from build123d import *

# Parameters (mm, degrees)
SKETCH2_R           = 17.5
SKETCH2_R_2         = 1.475
SKETCH2_R_3         = 4
BOSS_EXTRUDE1_DEPTH = 2.5
SKETCH3_R           = 7.5
SKETCH3_R_2         = 4
BOSS_EXTRUDE2_DEPTH = 10
FILLET1_R           = 1
SKETCH7_R           = 2.153442821
CUT_EXTRUDE7_DEPTH  = 5
CIRPATTERN2_COUNT   = 4


with BuildPart() as part:
    # Sketch2 → Boss-Extrude1 (new body)
    with BuildSketch(Plane(origin=(0, 0, 0), x_dir=(1, 0, 0), z_dir=(0, 1, 0))):
        with Locations(Location((0, 0, 0), (0, 0, 270))):
            Circle(SKETCH2_R)
        with Locations(Location((-12, 0, 0), (0, 0, 270))):
            Circle(SKETCH2_R_2, mode=Mode.SUBTRACT)
        with Locations(Location((0, -12, 0), (0, 0, 270))):
            Circle(SKETCH2_R_2, mode=Mode.SUBTRACT)
        with Locations(Location((12, 0, 0), (0, 0, 270))):
            Circle(SKETCH2_R_2, mode=Mode.SUBTRACT)
        with Locations(Location((0, 12, 0), (0, 0, 270))):
            Circle(SKETCH2_R_2, mode=Mode.SUBTRACT)
        with Locations(Location((0, 0, 0), (0, 0, 270))):
            Circle(SKETCH2_R_3, mode=Mode.SUBTRACT)
    extrude(amount=BOSS_EXTRUDE1_DEPTH)

    # Sketch3 → Boss-Extrude2 (add)
    with BuildSketch(Plane(origin=(0, 2.5, 0), x_dir=(1, 0, 0), z_dir=(0, 1, 0))):
        with Locations(Location((0, 0, 0), (0, 0, 270))):
            Circle(SKETCH3_R)
        with Locations(Location((0, 0, 0), (0, 0, 270))):
            Circle(SKETCH3_R_2, mode=Mode.SUBTRACT)
    extrude(amount=BOSS_EXTRUDE2_DEPTH)

    # Fillet1
    fillet1_edges = [part.edges().sort_by_distance(p)[0] for p in [
        (0, 12.5, -7.5),
    ]]
    fillet(fillet1_edges, radius=FILLET1_R)

    # Sketch7 → Cut-Extrude7 (cut)
    with BuildSketch(Plane(origin=(5.303300859, 0, 5.303300859), x_dir=(0, -1, 0), z_dir=(0.7071067811865464, 0, 0.7071067811865488))):
        with Locations(Location((-7, 0, 0), (0, 0, 90))):
            Circle(SKETCH7_R)
    cut_extrude7 = extrude(amount=-CUT_EXTRUDE7_DEPTH, mode=Mode.SUBTRACT)

    # CirPattern2: Cut-Extrude7 ×4 about axis
    cirpattern2_axis = Axis((0, 12.5, 0), (0, -1, 0))
    for i in range(1, CIRPATTERN2_COUNT):
        add(cut_extrude7.rotate(cirpattern2_axis, i * 360 / CIRPATTERN2_COUNT), mode=Mode.SUBTRACT)


solid = part.part
Check sheet for the modelled part. Datum: model origin and axes. Units: mm. A direction names the side the tool comes from. Give positions to 0.01 mm unless a question says otherwise; leave off trailing zeros. Loops run counter-clockwise (first coordinate to the right, second up) from the corner with the lowest first, then second, coordinate; pieces in that order, holes last. Notation, with made-up numbers: M 41.25,20.5 L 82.25,20.5 A4 cw 82.25,27.5 Z; hole C 15.5,-21.5 d1. An arc over 180 degrees is marked long. Return JSON: item names as keys, results as strings. Group by question number.
1. Cross-section at D-D on x = 13. Record the boundary of the cut face in (y, z).
2. Go/stop test with flat-tipped pins: pin 1 (6 mm diameter, centred on x = 11.5, z = -4.5, fed in from +Y); pin 2 (4 mm diameter, centred on x = 0, z = 12, fed in from -Y); pin 3 (6 mm diameter, centred on y = 5, z = -4.5, fed in from -X); pin 4 (5 mm diameter, centred on y = 8.5, z = -2, fed in from +X). Record where each tip stops, or that it passes through.
3. Cross-section at B-B on z = 0. Record the boundary of the cut face in (x, y) (3 decimals).
4. Cross-section at C-C on z = -11.5. Record the boundary of the cut face in (x, y).
5. Cross-section at A-A on x = 0. Record the boundary of the cut face in (y, z) (3 decimals).
6. Mould release check, pull along Z, two halves, no side actions. Record for faces 3 (the flat face through (3, 12.5, 3)), 4 (the cylindrical face through (-5.073, 5.69, 2.656)), 5 (the cylindrical face through (-10.648, 1.232, -13.887)): released by +Z, released by -Z, zero draft, split by the parting line, or undercut.
7. Tool access check on faces 1 (the flat face through (-8, 2.5, 0)), 2 (the cylindrical face through (13.244, 1.232, 0.793)). Record the directions out of +Z, -Z, +X, -X, +Y, -Y that give a thin tool (end or side, any length) a straight path to the whole face; none if there is none.
8. Thickness scan on L1, parallel to X at y = 0.6, z = 0 (3 decimals); L2, parallel to X at y = 4.5, z = 0; L3, parallel to Y at x = 10, z = 14. Record the ranges inside material, lowest first.
Return value:
{
 "1": {"outline": "M 0,-11.72 L 2.5,-11.72 L 2.5,-1.08 L 0,-1.08 Z; M 0,1.08 L 2.5,1.08 L 2.5,11.72 L 0,11.72 Z"},
 "2": {"pin 1": "y = 2.5", "pin 2": "y = 0", "pin 3": "x = -17.27", "pin 4": "x = 7.5"},
 "3": {"outline": "M -17.5,0 L -13.475,0 L -13.475,2.5 L -17.5,2.5 Z; M -10.525,0 L -4,0 L -4,12.5 L -6.5,12.5 A1 ccw -7.5,11.5 L -7.5,2.5 L -10.525,2.5 Z; M 4,0 L 10.525,0 L 10.525,2.5 L 7.5,2.5 L 7.5,11.5 A1 ccw 6.5,12.5 L 4,12.5 Z; M 13.475,0 L 17.5,0 L 17.5,2.5 L 13.475,2.5 Z"},
 "4": {"outline": "M -13.19,0 L -1.39,0 L -1.39,2.5 L -13.19,2.5 Z; M 1.39,0 L 13.19,0 L 13.19,2.5 L 1.39,2.5 Z"},
 "5": {"outline": "M 0,-17.5 L 2.5,-17.5 L 2.5,-13.475 L 0,-13.475 Z; M 0,-10.525 L 2.5,-10.525 L 2.5,-7.5 L 11.5,-7.5 A1 ccw 12.5,-6.5 L 12.5,-4 L 0,-4 Z; M 0,4 L 12.5,4 L 12.5,6.5 A1 ccw 11.5,7.5 L 2.5,7.5 L 2.5,10.525 L 0,10.525 Z; M 0,13.475 L 2.5,13.475 L 2.5,17.5 L 0,17.5 Z"},
 "6": {"face 3": "zero draft", "face 4": "undercut", "face 5": "split by the parting line"},
 "7": {"face 1": "+Y", "face 2": "+Y, -Y"},
 "8": {"L1": "-17.5 to -13.475, -10.525 to -4, 4 to 10.525, 13.475 to 17.5", "L2": "-7.5 to -4, 4 to 7.5", "L3": "0 to 2.5"}
}
